Can you work these out from the drawing? Everything is in mm from the part's minimum corner. A direction names the side the tool comes from. Give positions to 0.01 mm unless a question says otherwise; leave off trailing zeros. Write each loop counter-clockwise with the first axis right and the second up, starting at its lowest first coordinate (ties: lowest second). Pieces come first, ordered by that corner, then holes. Notation, with made-up numbers: (86, 36.25) -> (92, 36.25) arc R25 cw to (92, 70.25) -> close; hole circle Ø5 at (77.5, -3.75). An arc over 180 degrees is marked (long way). Return JSON: item names as keys, results as strings.
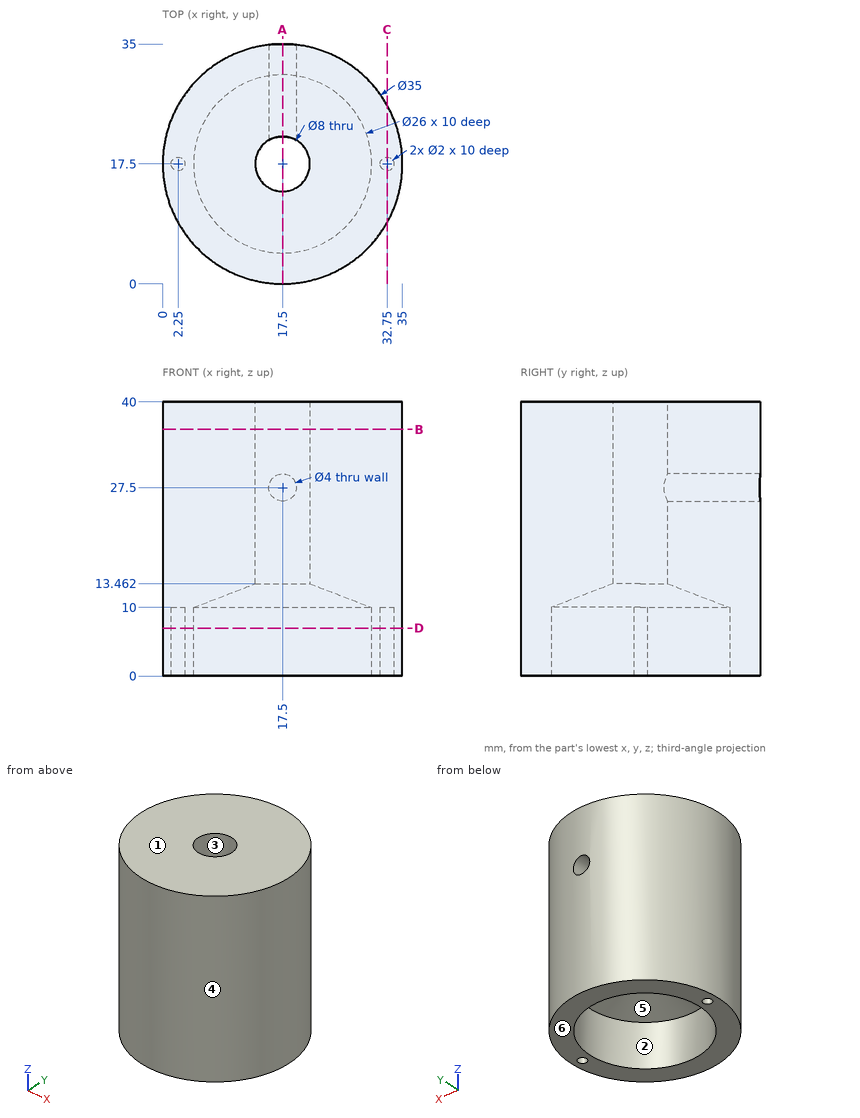
1. Suppose I cut it at D-D, the plane z = 7. List the corners of the cut face in (x, y) for me.
Taken from the geometry:
{"outline": "circle Ø35 at (17.5, 17.5); hole circle Ø2 at (2.25, 17.5); hole circle Ø26 at (17.5, 17.5); hole circle Ø2 at (32.75, 17.5)"}
2. Suppose I cut it at A-A, the plane x = 17.5. List the corners of the cut face in (y, z) for me, and give its area (3 significant figures).
Taken from the geometry:
{"outline": "(0, 0) -> (4.5, 0) -> (4.5, 10) -> (13.5, 13.46) -> (13.5, 40) -> (0, 40) -> close; (21.5, 13.46) -> (30.5, 10) -> (30.5, 0) -> (35, 0) -> (35, 25.5) -> (21.5, 25.5) -> close; (21.5, 29.5) -> (35, 29.5) -> (35, 40) -> (21.5, 40) -> close", "area": "815 mm²"}
3. For pin 1 Ø2 at (y, z) = (27, 35.5) entering from +X; pin 2 Ø4 at (y, z) = (13.5, 22.5) entering from -X (1 decimal); pin 3 Ø1.8 at (x, y) = (32.75, 17.5) entering from -Z, each with a flat end and sliding along its axis, tell me the tip position at first contact or that it passes through.
Taken from the geometry:
{"pin 1": "stops at x = 32.8", "pin 2": "stops at x = 0.1", "pin 3": "stops at z = 10"}
4. Suppose I cut it at C-C, the plane x = 32.75. List the corners of the cut face in (y, z) for me (1 decimal), and give its area (3 significant figures).
Taken from the geometry:
{"outline": "(8.9, 0) -> (16.5, 0) -> (16.5, 10) -> (18.5, 10) -> (18.5, 0) -> (26.1, 0) -> (26.1, 40) -> (8.9, 40) -> close", "area": "667 mm²"}
5. If we mould it in two halves opening along X, with no side actions, what happens to the marked faces 3, 4, 5 and 6? For each: released by +X, released by -X, zero draft, split by the parting line, or undercut.
Taken from the geometry:
{"face 3": "undercut", "face 4": "split by the parting line", "face 5": "undercut", "face 6": "zero draft"}
6. Which directions (+Z, -Z, +X, -X, +Y, -Y) give clear straight access to the entire face, cutting with the end or side of a thin tool? Please do the marked faces 1 and 2.
Taken from the geometry:
{"face 1": "+Z, +X, -X, +Y, -Y", "face 2": "-Z"}
7. If I drill on line 1 (X direction, y = 17, z = 6) (1 decimal); line 2 (X direction, y = 29, z = 2) (1 decimal); line 3 (X direction, y = 20, z = 33), over which ranges is the centre line in solid material (lowest first)? Write a range as [from, to].
Taken from the geometry:
{"line 1": "x = [0, 1.4], [3.1, 4.5], [30.5, 31.9], [33.6, 35]", "line 2": "x = [4.3, 11.4], [23.6, 30.7]", "line 3": "x = [0.18, 14.38], [20.62, 34.82]"}
8. Suppose I cut it at B-B, the plane z = 36. List the corners of the cut face in (x, y) for me.
Taken from the geometry:
{"outline": "circle Ø35 at (17.5, 17.5); hole circle Ø8 at (17.5, 17.5)"}
